Verification items for the finished model (mm, model axes). A direction names the side the tool comes from. Coordinates: 2 decimals unless noted, no trailing zeros. Order: outer loops, then holes, each group sorted by start corner. A loop starts at its lowest first (then second) coordinate and runs counter-clockwise, first axis right, second up. Notation, with made-up numbers: M 56,51.5 L 100,51.5 A32 cw 100,86.5 Z; hole C 75,-31.5 d3. An arc over 180 degrees is marked long. Return JSON: item names as keys, results as strings. Group by question number.
Q1. Section check C-C, the plane x = -5. Enter the section's corners in (y, z), then the cut area to 3 significant figures.
Q2. Section check A-A, the plane x = 4.5. Enter the section's corners in (y, z).
Q3. Thickness scan on probe 1 along Y at (x, z) = (-0.75, 0); probe 2 along X at (y, z) = (2.5, 0); probe 3 along X at (y, z) = (30, 6.25). Record the ranges inside material, lowest first.
Q4. Section check B-B, the plane y = 4. Enter the section's corners in (x, z), then the cut area to 3 significant figures.
Q5. Go/stop test with flat-tipped pins: pin 1 Ø1 at (y, z) = (31, 0.5) entering from +X; pin 2 Ø4 at (x, z) = (-4, -1) entering from +Y; pin 3 Ø1 at (y, z) = (29.5, 4) entering from -X; pin 4 Ø5 at (x, y) = (-5.5, 16) entering from -Z. Record where each tip stops, or that it passes through.
Q6. Mould release check, pull along X, two halves, no side actions. Record for faces 4 (the face through (1.88, 3.7, -5.96)), 5 (the face through (-4, 10, 0)), 6 (the face through (2.365, 32.49, 5.101)): pulls with the +X half, pulls with the -X half, needs draft (parallel to the pull), parting line crosses it, or undercut.
Q7. Access from +Z, -Z, +X, -X, +Y, -Y to the whole of each face (thin tool, end or side, straight path). Record for faces 1 (the face through (-2.5, 22, 0)), 2 (the face through (5, 10, 0)), 3 (the face through (0, 7.5, 0)).
from build123d import *

# Parameters (mm, degrees)
SKETCH1_R           = 7.5
BOSS_EXTRUDE1_DEPTH = 10
SKETCH2_R           = 6.25
CUT_EXTRUDE2_DEPTH  = 7.5
SKETCH3_W           = 5
SKETCH3_H           = 15
BOSS_EXTRUDE2_DEPTH = 25
SKETCH4_R           = 2.5
CUT_EXTRUDE3_DEPTH  = 5
FILLET1_R           = 7.5
CHAMFER1_SIZE       = 0.5


# Some blends are built 0.0001 mm under size
with BuildPart() as part:
    # Sketch1 → Boss-Extrude1 (new body)
    with BuildSketch(Plane(origin=(0, 0, 0), x_dir=(1, 0, 0), z_dir=(0, 1, 0))):
        with Locations(Location((0, 0, 0), (0, 0, 270))):
            Circle(SKETCH1_R)
    extrude(amount=BOSS_EXTRUDE1_DEPTH)

    # Sketch2 → Cut-Extrude2 (cut)
    with BuildSketch(Plane.XZ):
        with Locations(Location((0, 0, 0), (0, 0, 270))):
            Circle(SKETCH2_R)
    extrude(amount=-CUT_EXTRUDE2_DEPTH, mode=Mode.SUBTRACT)

    # Sketch3 → Boss-Extrude2 (add)
    with BuildSketch(Plane(origin=(0, 10, 0), x_dir=(1, 0, 0), z_dir=(0, 1, 0))):
        Rectangle(SKETCH3_W, SKETCH3_H)
    extrude(amount=BOSS_EXTRUDE2_DEPTH)

    # Sketch4 → Cut-Extrude3 (cut)
    with BuildSketch(Plane(origin=(2.5, 0, 0), x_dir=(0, 0, -1), z_dir=(1, 0, 0))):
        with Locations((0, 27.5)):
            Circle(SKETCH4_R)
    extrude(amount=-CUT_EXTRUDE3_DEPTH, mode=Mode.SUBTRACT)

    # Fillet1
    fillet1_edges = [part.edges().sort_by_distance(p)[0] for p in [
        (0, 35, -7.5),
        (0, 35, 7.5),
    ]]
    fillet(fillet1_edges, radius=FILLET1_R - 0.0001)  # a hair under: the kernel refuses the full size

    # Chamfer1
    # the kernel refuses this chamfer: 0.5 mm, written as the material it takes off along each edge
    with BuildSketch(Plane(origin=(-2.5, 10, 7.5), x_dir=(-0.027495876610586462, 0, -0.9996219169112968), z_dir=(0, 1, 0)), Plane(origin=(2.5, 10, 7.5), x_dir=(-0.9996219169112968, 0, 0.027495876610585623), z_dir=(0, 1, 0))) as chamfer1_piece_1:
        Polygon((CHAMFER1_SIZE * 0.999621916911, -CHAMFER1_SIZE * 0.0274958766106), (-CHAMFER1_SIZE * 0.0274958766106, -CHAMFER1_SIZE * 0.999621916911), (0, 0), align=None)
    extrude(amount=17.5001, mode=Mode.SUBTRACT)
    with BuildSketch(Plane(origin=(-2.5, 10, -7.5), x_dir=(-0.02749587661058651, 0, 0.9996219169112968), z_dir=(0, 1, 0)), Plane(origin=(2.5, 10, -7.5), x_dir=(-0.9996219169112968, 0, -0.027495876610585623), z_dir=(0, 1, 0))) as chamfer1_piece_2:
        Polygon((CHAMFER1_SIZE * 0.999621916911, CHAMFER1_SIZE * 0.0274958766106), (-CHAMFER1_SIZE * 0.0274958766106, CHAMFER1_SIZE * 0.999621916911), (0, 0), align=None)
    extrude(amount=17.5001, mode=Mode.SUBTRACT)
    with BuildSketch(Plane(origin=(-2.5, 27.5001, 0.0001), x_dir=(0, 0, 1), z_dir=(0, -1, 0))) as chamfer1_piece_3:
        Polygon((7.4999 - CHAMFER1_SIZE, 0), (7.4999, -CHAMFER1_SIZE), (7.4999, 0), align=None)
    revolve(axis=Axis((-2.5, 27.5001, 0.0001), (-1, 0, 0)), revolution_arc=90, mode=Mode.SUBTRACT)
    with BuildSketch(Plane(origin=(-2.5, 27.5001, -0.0001), x_dir=(0, 0, -1), z_dir=(0, -1, 0))) as chamfer1_piece_4:
        Polygon((7.4999 - CHAMFER1_SIZE, 0), (7.4999, CHAMFER1_SIZE), (7.4999, 0), align=None)
    revolve(axis=Axis((-2.5, 27.5001, -0.0001), (1, 0, 0)), revolution_arc=90, mode=Mode.SUBTRACT)
    with BuildSketch(Plane(origin=(2.5, 27.5001, 0.0001), x_dir=(0, 0, 1), z_dir=(0, -1, 0))) as chamfer1_piece_5:
        Polygon((7.4999, CHAMFER1_SIZE), (7.4999 - CHAMFER1_SIZE, 0), (7.4999, 0), align=None)
    revolve(axis=Axis((2.5, 27.5001, 0.0001), (-1, 0, 0)), revolution_arc=90, mode=Mode.SUBTRACT)
    with BuildSketch(Plane(origin=(2.5, 27.5001, -0.0001), x_dir=(0, 0, -1), z_dir=(0, -1, 0))) as chamfer1_piece_6:
        Polygon((7.4999, -CHAMFER1_SIZE), (7.4999 - CHAMFER1_SIZE, 0), (7.4999, 0), align=None)
    revolve(axis=Axis((2.5, 27.5001, -0.0001), (1, 0, 0)), revolution_arc=90, mode=Mode.SUBTRACT)
    with BuildSketch(Plane(origin=(2.5, 35, 0.0001), x_dir=(-0.999621916911297, 0.027495876610582174, 0), z_dir=(0, 0, -1))) as chamfer1_piece_7:
        Polygon((CHAMFER1_SIZE * 0.999621916911, -CHAMFER1_SIZE * 0.0274958766106), (-CHAMFER1_SIZE * 0.0274958766106, -CHAMFER1_SIZE * 0.999621916911), (0, 0), align=None)
    extrude(amount=0.0002, mode=Mode.SUBTRACT)
    with BuildSketch(Plane(origin=(-2.5, 35, -0.0001), x_dir=(-0.027495876610586605, -0.9996219169112968, 0), z_dir=(0, 0, 1))) as chamfer1_piece_8:
        Polygon((CHAMFER1_SIZE * 0.999621916911, CHAMFER1_SIZE * 0.0274958766106), (-CHAMFER1_SIZE * 0.0274958766106, CHAMFER1_SIZE * 0.999621916911), (0, 0), align=None)
    extrude(amount=0.0002, mode=Mode.SUBTRACT)


solid = part.part
Numbers:
{
 "1": {"outline": "M 0,-5.59 L 10,-5.59 L 10,5.59 L 0,5.59 L 0,3.75 L 7.5,3.75 L 7.5,-3.75 L 0,-3.75 Z", "area": "55.6 mm2"},
 "2": {"outline": "M 0,-6 L 10,-6 L 10,6 L 0,6 L 0,4.34 L 7.5,4.34 L 7.5,-4.34 L 0,-4.34 Z"},
 "3": {"probe 1": "y = 7.5 to 25, 30 to 35", "probe 2": "x = -7.5 to -6.25, 6.25 to 7.5", "probe 3": "x = -2.5 to 2.5"},
 "4": {"outline": "C 0,0 d15; hole C 0,0 d12.5", "area": "54.0 mm2"},
 "5": {"pin 1": "stops at x = 2.5", "pin 2": "stops at y = 34.95", "pin 3": "stops at x = -2.5", "pin 4": "passes through"},
 "6": {"face 4": "undercut", "face 5": "needs draft", "face 6": "pulls with the +X half"},
 "7": {"face 1": "+Z, -Z, -X, +Y", "face 2": "+Z, -Z, +X, +Y", "face 3": "-Y"}
}
